```python
from build123d import *

# Parameters (mm, degrees)
SKETCH_W        = 40
SKETCH_H        = 85
PAD_DEPTH       = 10
SKETCH001_R     = 2.4
POCKET_DEPTH    = 10
SKETCH002_R     = 5
POCKET001_DEPTH = 5


with BuildPart() as part:
    # Sketch → Pad (new body)
    with BuildSketch(Plane.XZ):
        Rectangle(SKETCH_W, SKETCH_H)
    extrude(amount=PAD_DEPTH)

    # Sketch001 (on Face6 of Pad) → Pocket (cut)
    with BuildSketch(Plane.XZ.offset(10)):
        with Locations((-10, -32.5)):
            Circle(SKETCH001_R)
        with Locations((10, -32.5)):
            Circle(SKETCH001_R)
        with Locations((10, 32.5)):
            Circle(SKETCH001_R)
        with Locations((10, 17.5)):
            Circle(SKETCH001_R)
    extrude(amount=-POCKET_DEPTH, mode=Mode.SUBTRACT)

    # Sketch002 (on Face5 of Pocket) → Pocket001 (cut)
    with BuildSketch(Plane.XZ.offset(10)):
        with Locations((-10, -32.5)):
            Circle(SKETCH002_R)
        with Locations((10, -32.5)):
            Circle(SKETCH002_R)
        Polygon((13.897114, 30.25), (13.897114, 34.75), (10, 37), (6.102886, 34.75), (6.102886, 30.25), (10, 28), align=None)
        Polygon((13.897114, 15.25), (13.897114, 19.75), (10, 22), (6.102886, 19.75), (6.102886, 15.25), (10, 13), align=None)
    extrude(amount=-POCKET001_DEPTH, mode=Mode.SUBTRACT)


solid = part.part
```
Geometry check sheet. Reference: the model listing, model coordinates, mm. A direction names the side the tool comes from. Coordinates: 2 decimals unless noted, no trailing zeros. Order: outer loops, then holes, each group sorted by start corner. A loop starts at its lowest first (then second) coordinate and runs counter-clockwise, first axis right, second up.
Q1. Sectioned sample at D-D on y = -2.5. Record the cut outline in (x, z).
Reply:
outline: (-20, -42.5) - (20, -42.5) - (20, 42.5) - (-20, 42.5) - close; hole circle Ø4.8 at (-10, -32.5); hole circle Ø4.8 at (10, -32.5); hole circle Ø4.8 at (10, 17.5); hole circle Ø4.8 at (10, 32.5)
Q2. Depth check by flat-ended pin: pin 1 Ø5 at (x, z) = (11.5, -31) entering from -Y. Enter the tip coordinate at first touch or a pass-through.
Reply:
pin 1: stops at y = -5
Q3. Draft check along Z on faces 3 (the face through (9.48, -2.535, 15.157)), 4 (the face through (20, -5, -1)), 5 (the face through (9.48, -2.535, 30.157)), 6 (the face through (0, -5, 42.5)). Enter one of: released by +Z, released by -Z, zero draft, split by the parting line, or undercut.
Reply:
face 3: undercut
face 4: zero draft
face 5: undercut
face 6: released by +Z
Q4. Thickness scan on probe 1 along Z at (x, y) = (10, -1.6); probe 2 along Z at (x, y) = (10, -6.55); probe 3 along X at (y, z) = (-6.75, 20). Record the ranges inside material, lowest first.
Reply:
probe 1: z = -42.5 to -34.9, -30.1 to 15.1, 19.9 to 30.1, 34.9 to 42.5
probe 2: z = -42.5 to -37.5, -27.5 to 13, 22 to 28, 37 to 42.5
probe 3: x = -20 to 6.54, 13.46 to 20
Q5. Tool access check on faces 1 (the face through (-10.52, -2.535, -34.843)), 2 (the face through (6.103, -8, 33)). Record the directions out of +Z, -Z, +X, -X, +Y, -Y that give a thin tool (end or side, any length) a straight path to the whole face; none if there is none.
Reply:
face 1: +Y, -Y
face 2: -Y
Q6. Sectioned sample at B-B on x = -10. Record the cut outline in (y, z), and give its area (3 significant figures).
Reply:
outline: (-10, -42.5) - (0, -42.5) - (0, -34.9) - (-5, -34.9) - (-5, -37.5) - (-10, -37.5) - close; (-10, -27.5) - (-5, -27.5) - (-5, -30.1) - (0, -30.1) - (0, 42.5) - (-10, 42.5) - close
area: 776 mm2
Q7. Sectioned sample at C-C on z = -32.5. Record the cut outline in (x, y), and give its area (3 significant figures).
Reply:
outline: (-20, -10) - (-15, -10) - (-15, -5) - (-12.4, -5) - (-12.4, 0) - (-20, 0) - close; (-7.6, -5) - (-5, -5) - (-5, -10) - (5, -10) - (5, -5) - (7.6, -5) - (7.6, 0) - (-7.6, 0) - close; (12.4, -5) - (15, -5) - (15, -10) - (20, -10) - (20, 0) - (12.4, 0) - close
area: 252 mm2
Q8. Sectioned sample at A-A on z = 17.5. Record the cut outline in (x, y), and give its area (3 significant figures).
Reply:
outline: (-20, -10) - (6.1, -10) - (6.1, -5) - (7.6, -5) - (7.6, 0) - (-20, 0) - close; (12.4, -5) - (13.9, -5) - (13.9, -10) - (20, -10) - (20, 0) - (12.4, 0) - close
area: 337 mm2
